Input: dimensioned drawing with shaded views. Units: mm. Origin: part minimum x, y, z. A direction names the side the tool comes from. Round coordinates to 2 decimals unless told otherwise and drop trailing zeros. Loops run counter-clockwise (first coordinate to the right, second up) from the corner with the lowest first, then second, coordinate; pieces in that order, holes last. Notation, with made-up numbers: (50, 41.5) - (90, 41.5) arc R6 cw to (90, 52.5) - close; hole circle Ø1 at (-6.5, 35). An arc over 180 degrees is marked (long way). Answer as a JSON object with one key per item and string values. Group by question number.
Item 1: Line query: line 1 (X direction, y = 9.4, z = 7); line 2 (X direction, y = 1.3, z = 7); line 3 (Y direction, x = 1.25, z = 6). Output: solid intervals per line, ascending.
Item 2: Draft query along X for the marked faces 3, 4 and 5. Return one class per face: released by +X, released by -X, zero draft, split by the parting line, or undercut.
Item 3: Reachability of the marked faces 1 and 2 from +Z, -Z, +X, -X, +Y, -Y: full face, straight path, thin tool, end or side. Return the list, or none.
Item 4: Section C-C (y = 9.25). Return the cut outline in (x, z).
Item 5: First-contact query: pin 1 (2 mm diameter, centred on x = 5.5, z = 5.5, fed in from -Y); pin 2 (1.3 mm diameter, centred on x = 8, z = 7.5, fed in from +Y); pin 3 (2 mm diameter, centred on x = 11.5, y = 6.5, fed in from -Z). Flat tips, straight axial feed; report the tip coordinate or a pass-through.
Item 6: Section D-D (y = 5.75). Return the cut outline in (x, z).
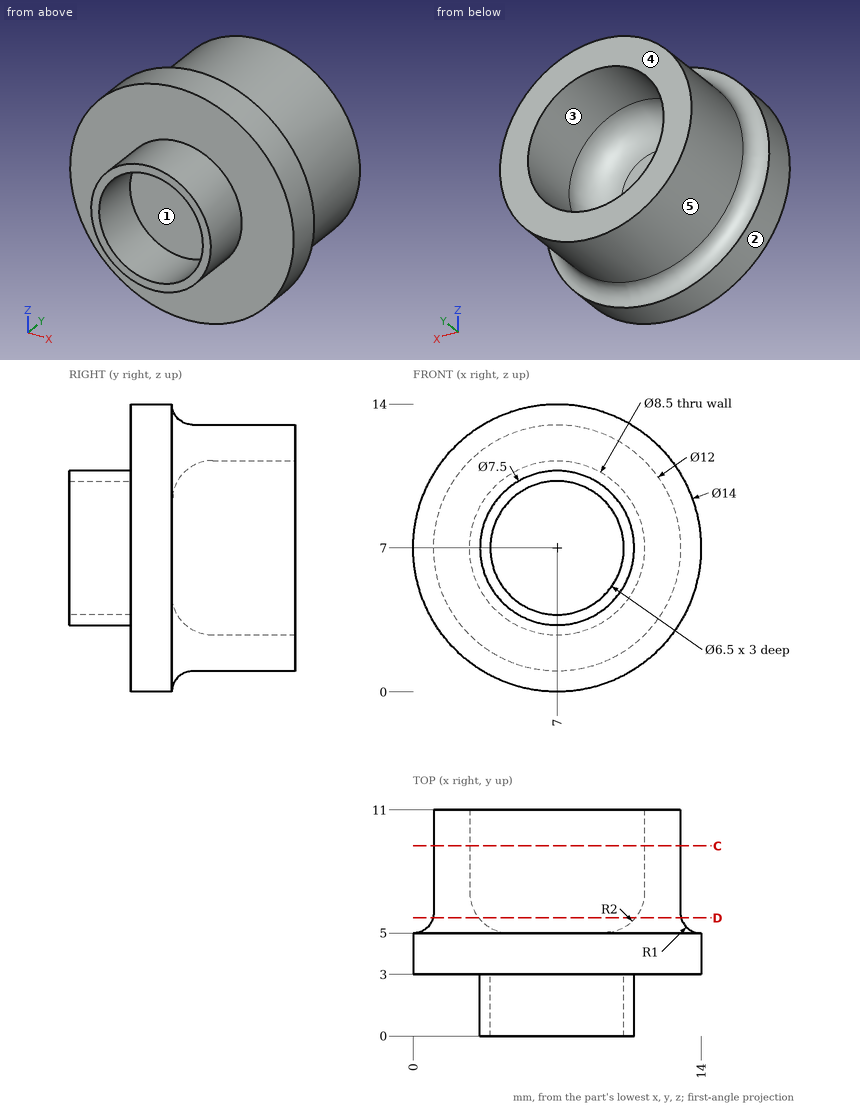
Values:
{
 "1": {"line 1": "x = 1 to 2.75, 11.25 to 13", "line 2": "x = 3.25 to 3.75, 10.25 to 10.75", "line 3": "y = 3 to 11"},
 "2": {"face 3": "undercut", "face 4": "zero draft", "face 5": "split by the parting line"},
 "3": {"face 1": "-Y", "face 2": "+Y, -Y"},
 "4": {"outline": "circle Ø12 at (7, 7); hole circle Ø8.5 at (7, 7)"},
 "5": {"pin 1": "stops at y = 3", "pin 2": "stops at y = 5", "pin 3": "stops at z = 2.13"},
 "6": {"outline": "circle Ø12.06 at (7, 7); hole circle Ø7.62 at (7, 7)"}
}
